The model under review builds one solid part; all positions refer to its coordinate system, in mm. A direction names the side the tool comes from. Give positions to 0.01 mm unless a question says otherwise; leave off trailing zeros. Loops run counter-clockwise (first coordinate to the right, second up) from the corner with the lowest first, then second, coordinate; pieces in that order, holes last. Notation, with made-up numbers: (82, -15) - (103, -15) arc R33 cw to (103, 22) - close; hole circle Ø7 at (48, -6). An arc over 180 degrees is marked (long way). Return JSON: item names as keys, results as strings. Group by question number.
```python
from build123d import *

# Parameters (mm, degrees)
F1_DEPTH    = 10
F2_T1_DEPTH = 10
F2_T3_DEPTH = 21
F2_T5_DEPTH = 21
F3_W        = 3
F3_H        = 5
F4_DEPTH    = 25
F5_R        = 1


# Not quite as in the source:
# - a fillet or chamfer that OpenCascade refuses, or shapes differently, is made with other operations: its cross-section is extruded or revolved along the edge and cut away or added


with BuildPart() as f1:
    # F0 (on Right) → F1 (new body)
    with BuildSketch(Plane.YZ):
        with BuildLine():
            Line((0, 2.5), (0, 0))
            Line((0, 0), (34, 0))
            Line((34, 0), (34, 6))
            Line((34, 6), (19, 6))
            Line((19, 6), (19, 8.927215822))
            add(Edge.make_bspline(
                [(13.5019160807, 15.3781203553), (14.3536763756, 15.0835294533), (15.3076259705, 14.7454615797), (17.8235832578, 12.8012966962), (18.7947445626, 9.9588259689), (18.9257892428, 9.3615105358), (19, 8.927215822)],
                knots=[0, 0, 0, 0, 0.0707143844, 0.1572524963, 0.2414371446, 0.2933722159, 0.2933722159, 0.2933722159, 0.2933722159], degree=3))
            Line((13.5019160807, 15.3781203553), (5.3910082206, 15.3781203553))
            Line((5.3910082206, 15.3781203553), (5.3910082206, 13.2812492201))
            Line((5.3910082206, 13.2812492201), (5.3910082206, 11.7001235485))
            Line((5.3910082206, 11.7001235485), (9, 11.7001235485))
            ThreePointArc((9, 11.7001235485), (12.8276697655, 7.5089175953), (9, 3.317711642))
            Line((9, 3.317711642), (0, 2.5))
        make_face()
    extrude(amount=F1_DEPTH)

    # F2: fillet of radius 3 on 3 edges, made by hand

    # F2_s2 → F2_t1 (join)
    with BuildSketch(Plane.YZ):
        with BuildLine():
            ThreePointArc((19, 8.927215822), (19.9036876994, 6.8531007786), (21.9991169473, 6))
            Line((21.9991169473, 6), (19, 6))
            Line((19, 6), (19, 8.927215822))
        make_face()
    extrude(amount=F2_T1_DEPTH)

    # F2_s4 → F2_t3 (cut)
    with BuildSketch(Plane.XY.offset(-7.5)):
        with BuildLine():
            ThreePointArc((10, 31), (9.1213203436, 33.1213203436), (7, 34))
            Line((7, 34), (10, 34))
            Line((10, 34), (10, 31))
        make_face()
    extrude(amount=F2_T3_DEPTH, mode=Mode.SUBTRACT)

    # F2_s6 → F2_t5 (cut)
    with BuildSketch(Plane.XY.offset(-7.5)):
        with BuildLine():
            ThreePointArc((0, 31), (0.8786796564, 33.1213203436), (3, 34))
            Line((3, 34), (0, 34))
            Line((0, 34), (0, 31))
        make_face()
    extrude(amount=F2_T5_DEPTH, mode=Mode.SUBTRACT)

    # F3 (on face) → F4 (cut)
    with BuildSketch(Plane.XY.offset(6)):
        with Locations((5, 29.0757007897)):
            Rectangle(F3_W, F3_H)
    extrude(amount=-F4_DEPTH, mode=Mode.SUBTRACT)

    # F5
    f5_edges = [f1.edges().sort_by_distance(p)[0] for p in [
        (3.5, 26.575701, 3),
        (3.5, 31.575701, 3),
        (6.5, 26.575701, 3),
        (6.5, 31.575701, 3),
    ]]
    fillet(f5_edges, radius=F5_R)


solid = f1.part
```
1) We need section D-D, the plane z = 4.25. Write out the cut boundary in (x, y).
2) We need section C-C, the plane y = 6. Write out the cut boundary in (x, z).
3) Draft analysis for pull direction Z (two halves, no side actions). For faces 4 (the face through (6.215, 26.876, 2.958)), 5 (the face through (4.93, 4.563, 2.915)), 6 (the face through (3, 28, 6)), state which applies: +Z half, -Z half, draft (parallel to the pull), parting line (faces both ways), or undercut.
4) To check wall thickness, follow line 1 (X direction, y = 29, z = 4); line 2 (Z direction, x = 3.5, y = 5.5); line 3 (Z direction, x = 5, y = 22). State the ranges of each line that lie inside material, in increasing order.
5) For pin 1 Ø0.8 at (x, z) = (5, 4.5) entering from -Y; pin 2 Ø1.8 at (x, z) = (2.5, 13) entering from -Y; pin 3 Ø3 at (x, y) = (7, 25.5) entering from +Z, all flat-tipped, find the tip position at first contact; note any pin that passes through.
6) We need section B-B, the plane y = 11. Write out the cut boundary in (x, z).
7) Tool access review of faces 1 (the face through (5, 17, 0)), 2 (the face through (5, 7, 11.7)), 3 (the face through (5, 31.576, 3)): name each direction out of +Z, -Z, +X, -X, +Y, -Y from which nothing blocks a thin tool from reaching the whole face with its end or side.
8) We need section A-A, the plane z = 1.75. Write out the cut boundary in (x, y).
Findings:
{
 "1": {"outline": "(0, 11.28) - (10, 11.28) - (10, 31) arc R3 ccw to (7, 34) - (3, 34) arc R3 ccw to (0, 31) - close; hole (3.5, 27.58) arc R1 ccw to (4.5, 26.58) - (5.5, 26.58) arc R1 ccw to (6.5, 27.58) - (6.5, 30.58) arc R1 ccw to (5.5, 31.58) - (4.5, 31.58) arc R1 ccw to (3.5, 30.58) - close"},
 "2": {"outline": "(0, 0) - (10, 0) - (10, 3.05) - (0, 3.05) - close; (0, 11.7) - (10, 11.7) - (10, 15.38) - (0, 15.38) - close"},
 "3": {"face 4": "draft", "face 5": "undercut", "face 6": "+Z half"},
 "4": {"line 1": "x = 0 to 3.5, 6.5 to 10", "line 2": "z = 0 to 3, 11.7 to 15.38", "line 3": "z = 0 to 6"},
 "5": {"pin 1": "stops at y = 11.09", "pin 2": "stops at y = 5.39", "pin 3": "stops at z = 6"},
 "6": {"outline": "(0, 0) - (10, 0) - (10, 4.04) - (0, 4.04) - close; (0, 10.98) - (10, 10.98) - (10, 15.38) - (0, 15.38) - close"},
 "7": {"face 1": "-Z, +X, -X, +Y, -Y", "face 2": "+X, -X, -Y", "face 3": "+Z, -Z"},
 "8": {"outline": "(0, 0) - (10, 0) - (10, 31) arc R3 ccw to (7, 34) - (3, 34) arc R3 ccw to (0, 31) - close; hole (3.5, 27.58) arc R1 ccw to (4.5, 26.58) - (5.5, 26.58) arc R1 ccw to (6.5, 27.58) - (6.5, 30.58) arc R1 ccw to (5.5, 31.58) - (4.5, 31.58) arc R1 ccw to (3.5, 30.58) - close"}
}
